The listing builds one solid part. Answer for the finished solid, in the listing's coordinates (mm). Face numbers are marked on the shaded views. A direction names the side the tool comes from. Give positions to 0.01 mm unless a question says otherwise; leave off trailing zeros. Write each loop counter-clockwise with the first axis right and the second up, starting at its lowest first coordinate (ties: lowest second). Pieces come first, ordered by that corner, then holes. Notation, with made-up numbers: (53.25, -36) - (62.25, -36) arc R24 ccw to (62.25, 2) - close; hole circle Ø8 at (28.5, 89.25). An arc over 180 degrees is marked (long way). One line per question, with ' | ' between items. Start each with the question number.
1. For the marked faces 1, 2 and 3, determine the directions among +Z, -Z, +X, -X, +Y, -Y from which every point of the face is accessible in a straight line to the end or side of a thin tool.
2. A cutting plane is placed at A-A (y = 7). Determine the outline of the cut face in (x, z).
3. A cutting plane is placed at C-C (z = 3.25). Determine the outline of the cut face in (x, y), then the cut area to 3 significant figures.
4. Given P1, Ø1.5, axis at y = 24, z = 7.5, coming from the +X side; P2, Ø6, axis at x = 59.5, y = 18.5, coming from the -Z side; P3, Ø1.5, axis at x = 49.5, y = 19, coming from the +Z side; P4, Ø8.5, axis at x = 47.5, y = 7.5, coming from the -Z side, each flat-ended and moving along its own axis, determine where each tip first touches the part or whether it passes through.
5. A cutting plane is placed at B-B (z = 16.25). Determine the outline of the cut face in (x, y).
6. The mould has two halves that part along Z. Classify the marked faces 4, 5 and 6: +Z half, -Z half, draft (parallel to the pull), parting line (faces both ways), or undercut.
7. Find the intervals of material crossed by L1, parallel to Y at x = 50.5, z = 13.5; L2, parallel to X at y = 17, z = 2.75; L3, parallel to Y at x = 38.5, z = 5.75, in increasing order. Write a range as from..to.
8. A cutting plane is placed at D-D (y = 21.5). Determine the outline of the cut face in (x, z).
```python
from build123d import *

# Parameters (mm, degrees)
BOSS_EXTRUDE1_DEPTH = 10
SCALE1_SCALE        = 0.5
SKETCH4_W           = 2.5
SKETCH4_H           = 5
BOSS_EXTRUDE4_DEPTH = 12
SKETCH5_W           = 5
SKETCH5_H           = 10
BOSS_EXTRUDE5_DEPTH = 0.5
BOSS_EXTRUDE6_REACH = 83.657
SKETCH7_W           = 5
SKETCH7_H           = 7.071067812
SKETCH8_W           = 5
SKETCH8_H           = 1.464466094
SKETCH8_H_2         = 7.071067812
BOSS_EXTRUDE7_DEPTH = 12
FILLET1_START       = 49
FILLET1_DEPTH       = 7
FILLET1_START_2     = 50.028561354
FILLET1_2_DEPTH     = 5
CUT_EXTRUDE1_DEPTH  = 53.473637274
FILLET2_R           = 1


with BuildPart() as part:
    # Sketch1 → Boss-Extrude1 (new body)
    with BuildSketch(Plane.XY):
        with BuildLine():
            Line((0, 0), (5, 0))
            ThreePointArc((5, 0), (52.528561354, 12.453541306), (100.057122708, 0))
            Line((100.057122708, 0), (105.057122708, 0))
            ThreePointArc((105.057122708, 0), (52.528561354, 15.847728612), (0, 0))
        make_face()
    extrude(amount=BOSS_EXTRUDE1_DEPTH)


with BuildPart() as part_1:
    # Scale1: scaled about (52.528561354, 9.724546383, 5)
    add(part.part.scale(SCALE1_SCALE).moved(Location((26.264280677, 4.862273191, 2.5))))



with BuildPart() as body_2:
    # Sketch4 → Boss-Extrude4 (new body)
    with BuildSketch(Plane(origin=(0, 12.786137497, 0), x_dir=(1, 0, 0), z_dir=(0, 1, 0))):
        with Locations((53.778561354, -5)):
            Rectangle(SKETCH4_W, SKETCH4_H)
        Polygon((50.028561354, 0), (50.028561354, -2.5), (52.528561354, -2.5), (55.028561354, -2.5), (55.028561354, 0), align=None)
        with Locations((51.278561354, -5)):
            Rectangle(SKETCH4_W, SKETCH4_H)
        Polygon((52.528561354, -7.5), (50.028561354, -7.5), (50.028561354, -10), (55.028561354, -10), (55.028561354, -7.5), align=None)
    extrude(amount=BOSS_EXTRUDE4_DEPTH)


with BuildPart() as part_2:
    add(part_1.part)

    add(body_2.part)  # Boss-Extrude5 merges body 2
    # Sketch5 → Boss-Extrude5 (add)
    with BuildSketch(Plane.XZ.offset(-12.786137497)):
        with Locations((52.528561354, 5)):
            Rectangle(SKETCH5_W, SKETCH5_H)
    extrude(amount=BOSS_EXTRUDE5_DEPTH)

    # Boss-Extrude6: up to this plane
    boss_extrude6_end = Plane(origin=(50.028561354, 12.286137497, 0), z_dir=(0, 0, 1))
    # Sketch7 → Boss-Extrude6 (add, up to the surface)
    with BuildSketch(Plane(origin=(0, 17.393068749, 17.393068749), x_dir=(1, 0, 0), z_dir=(0, 0.7071067811865464, 0.7071067811865488)), mode=Mode.PRIVATE) as boss_extrude6_sk1:
        with Locations((52.528561354, 13.990911998)):
            Rectangle(SKETCH7_W, SKETCH7_H)
    boss_extrude6_tool1 = split(extrude(boss_extrude6_sk1.sketch, amount=-BOSS_EXTRUDE6_REACH, mode=Mode.PRIVATE), bisect_by=boss_extrude6_end, keep=Keep.BOTH, mode=Mode.PRIVATE)
    add(boss_extrude6_tool1.solids().sort_by_distance((52.528561, 27.286137, 7.5))[0])

    # Sketch8 → Boss-Extrude7 (add)
    with BuildSketch(Plane(origin=(0, 17.393068749, 17.393068749), x_dir=(1, 0, 0), z_dir=(0, 0.7071067811865465, 0.7071067811865487))):
        with Locations((52.528561354, 18.258678951)):
            Rectangle(SKETCH8_W, SKETCH8_H)
        with Locations((52.528561354, 13.990911998)):
            Rectangle(SKETCH8_W, SKETCH8_H_2)
        with Locations((52.528561354, 9.723145045)):
            Rectangle(SKETCH8_W, SKETCH8_H)
    extrude(amount=BOSS_EXTRUDE7_DEPTH)

    # Fillet1: read off the stored shape, not the designer's step
    # Fillet1 outline → Fillet1 (cut)
    with BuildSketch(Plane.YZ.offset(FILLET1_START)):
        with BuildLine():
            Line((23.750603591, 11.035533906), (24.786137497, 10))
            ThreePointArc((24.786137497, 10), (25.785055254, 12.542376711), (27.434667987, 14.719598301))
            Line((27.434667987, 14.719598301), (23.750603591, 11.035533906))
        make_face()
    extrude(amount=FILLET1_DEPTH, mode=Mode.SUBTRACT)

    # Fillet1 2 outline → Fillet1 2 (add)
    with BuildSketch(Plane.YZ.offset(FILLET1_START_2)):
        with BuildLine():
            Line((29.786137497, 5), (26.102073102, 1.315935604))
            ThreePointArc((26.102073102, 1.315935604), (28.279294693, 2.965548337), (30.821671403, 3.964466094))
            Line((30.821671403, 3.964466094), (29.786137497, 5))
        make_face()
    extrude(amount=FILLET1_2_DEPTH)

    # Sketch9 → Cut-Extrude1 (cut, through all)
    with BuildSketch(Plane(origin=(55.028561354, 0, 0), x_dir=(0, 0, -1), z_dir=(1, 0, 0))):
        Polygon((-12.980077554, 37.362409129), (-17.576271632, 32.766215052), (-13.333630945, 28.523574364), (-8.737436867, 33.119768442), align=None)
    extrude(amount=-CUT_EXTRUDE1_DEPTH, mode=Mode.SUBTRACT)

    # Fillet2
    fillet2_edges = [part_2.edges().sort_by_distance(p)[0] for p in [
        (52.528561354, 12.286137497, 2.5),
        (55.028561354, 12.503212632, 2.5),
        (50.028561354, 12.503212632, 2.5),
        (50.028561354, 12.503212632, 7.5),
        (55.028561354, 12.503212632, 7.5),
        (52.528561354, 12.286137497, 10),
        (52.528561354, 12.286137497, 7.5),
        (52.528561354, 12.286137497, 0),
    ]]
    fillet(fillet2_edges, radius=FILLET2_R)


solid = part_2.part
```
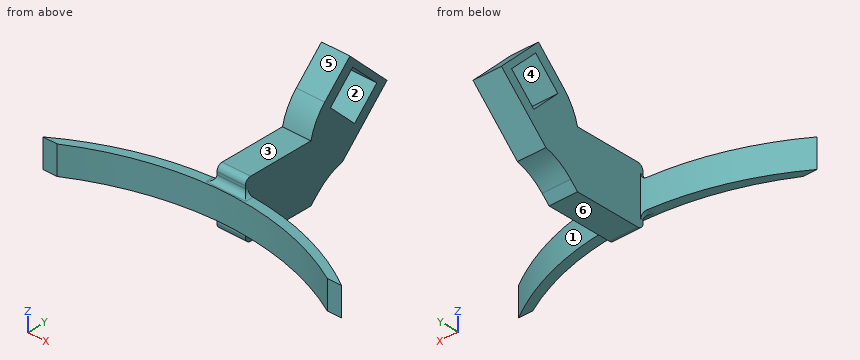
Determined:
1) face 1: +Z, -Z, +X, +Y | face 2: +X, -X | face 3: +Z, +X, -X, -Y
2) outline: (29.81, 2.5) - (33.05, 2.5) - (33.05, 7.5) - (29.81, 7.5) - close; (72.01, 2.5) - (75.25, 2.5) - (75.25, 7.5) - (72.01, 7.5) - close
3) outline: (26.26, 4.86) - (28.76, 4.86) arc R48.46 cw to (76.29, 4.86) - (78.79, 4.86) arc R47.49 ccw to (55.03, 12.72) - (55.03, 28.82) - (50.03, 28.82) - (50.03, 12.72) arc R47.49 ccw to start | area: 163 mm2
4) P1: x = 55.03 | P2: through | P3: z = 10 | P4: z = 2.49
5) outline: (50.03, 28.97) - (55.03, 28.97) - (55.03, 31.44) - (50.03, 31.44) - close; (50.03, 34.09) - (55.03, 34.09) - (55.03, 35.51) - (50.03, 35.51) - close
6) face 4: undercut | face 5: +Z half | face 6: -Z half
7) L1: 26.4..28.69, 36.84..38.26 | L2: 50.03..55.03 | L3: 9.01..10.67
8) outline: (50.03, 0) - (55.03, 0) - (55.03, 10) - (50.03, 10) - close
